Build history of the part. All positions in model axes, mm. Coordinates: 2 decimals unless noted, no trailing zeros. Write each loop counter-clockwise with the first axis right and the second up, starting at its lowest first coordinate (ties: lowest second). Pieces come first, ordered by that corner, then holes.
```python
from build123d import *

# Parameters (mm, degrees)
SKETCH9_3_W         = 12
SKETCH9_3_H         = 1
BOSS_EXTRUDE3_DEPTH = 4.5


with BuildPart() as part:
    # Sketch9_3 → Boss-Extrude3 (new body)
    with BuildSketch(Plane.XY):
        with BuildLine():
            Line((-5.979130372, -0.5), (-6, -0.5))
            Line((-6, -0.5), (-6, -8))
            Line((-6, -8), (6, -8))
            Line((6, -8), (6, -0.5))
            Line((6, -0.5), (5.979130372, -0.5))
            ThreePointArc((5.979130372, -0.5), (0, -6), (-5.979130372, -0.5))
        make_face()
        with Locations((0, -8.5)):
            Rectangle(SKETCH9_3_W, SKETCH9_3_H)
    extrude(amount=BOSS_EXTRUDE3_DEPTH)


solid = part.part
```
1. Saw through at C-C on x = -4.75. List the corners of the cut face in (y, z).
Computed values:
outline: (-9, 0) - (-3.67, 0) - (-3.67, 4.5) - (-9, 4.5) - close
2. Mould opens along X. For faces 1 (the face through (0, -6, 2)), 2 (the face through (-6, -5, 2)), 3 (the face through (0, -7, 0)), 4 (the face through (6, -5, 2)) say: +X half, -X half, draft (parallel to the pull), parting line (faces both ways), or undercut.
Computed values:
face 1: undercut
face 2: -X half
face 3: draft
face 4: +X half
3. Saw through at A-A on y = -4.75. List the corners of the cut face in (x, z), plus the area to 3 significant figures.
Computed values:
outline: (-6, 0) - (-3.67, 0) - (-3.67, 4.5) - (-6, 4.5) - close; (3.67, 0) - (6, 0) - (6, 4.5) - (3.67, 4.5) - close
area: 21.0 mm2
4. Saw through at D-D on y = -2.5. List the corners of the cut face in (x, z), plus the area to 3 significant figures.
Computed values:
outline: (-6, 0) - (-5.45, 0) - (-5.45, 4.5) - (-6, 4.5) - close; (5.45, 0) - (6, 0) - (6, 4.5) - (5.45, 4.5) - close
area: 4.91 mm2
5. Probe line 1 along Y through (x, z) = (0.5, 4.1); line 2 along X through (y, z) = (-2, 1.55); line 3 along X through (y, z) = (-1.5, 3). List the from-to ranges inside material, lowest first.
Computed values:
line 1: y = -9 to -5.98
line 2: x = -6 to -5.66, 5.66 to 6
line 3: x = -6 to -5.81, 5.81 to 6
